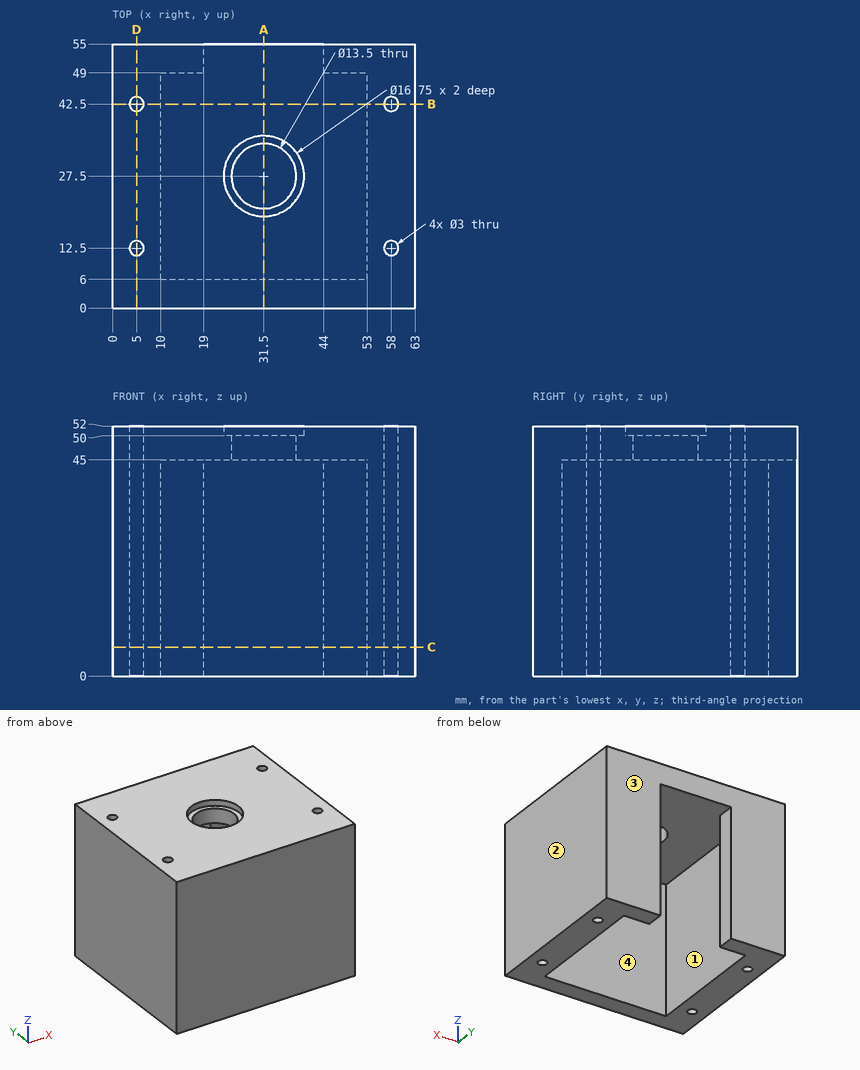
Here's the drawing with two shaded views (mm, measured from the low corner). I have some questions. Round coordinates to 2 decimals unless told otherwise and drop trailing zeros. Order: outer loops, then holes, each group sorted by start corner. A loop starts at its lowest first (then second) coordinate and runs counter-clockwise, first axis right, second up. Notation, with made-up numbers: (25, 72.5) -> (69, 72.5) arc R24 cw to (69, 109.5) -> close; hole circle Ø7 at (43, 34). An arc over 180 degrees is marked (long way). Use a Markdown table: item, result. Add a question column.
(1) Suppose I cut it at D-D, the plane x = 5. Please give me the cut outline in (y, z).
(2) Suppose I cut it at A-A, the plane x = 31.5. Please give me the cut outline in (y, z) (3 decimals).
(3) Suppose I cut it at B-B, the plane y = 42.5. Please give me the cut outline in (x, z).
(4) If we mould it in two halves opening along Y, with no side actions, what happens to the marked faces 1, 2, 3 and 4? For each: released by +Y, released by -Y, zero draft, split by the parting line, or undercut.
(5) For pin 1 Ø3.5 at (x, y) = (5, 42.5) entering from -Z; pin 2 Ø1.5 at (x, z) = (25, 36) entering from +Y; pin 3 Ø2.5 at (x, y) = (58, 12.5) entering from +Z; pin 4 Ø1.5 at (x, y) = (47, 11.5) entering from -Z, each with a flat end and sliding along its axis, tell me the tip position at first contact or that it passes through.
(6) I need wall thicknesses on line 1 along Y through (x, z) = (5, 19); line 2 along Y through (x, z) = (13.5, 24); line 3 along X through (y, z) = (48, 12). Which ranges of each line are inside material? Lowest first, please.
(7) Suppose I cut it at C-C, the plane z = 6. Please give me the cut outline in (x, y).
Verdict:
| question | item | result |
|---|---|---|
| 1 | outline | (0, 0) -> (11, 0) -> (11, 52) -> (0, 52) -> close; (14, 0) -> (41, 0) -> (41, 52) -> (14, 52) -> close; (44, 0) -> (55, 0) -> (55, 52) -> (44, 52) -> close |
| 2 | outline | (0, 0) -> (6, 0) -> (6, 45) -> (20.75, 45) -> (20.75, 50) -> (19.125, 50) -> (19.125, 52) -> (0, 52) -> close; (34.25, 45) -> (55, 45) -> (55, 52) -> (35.875, 52) -> (35.875, 50) -> (34.25, 50) -> close |
| 3 | outline | (0, 0) -> (3.5, 0) -> (3.5, 52) -> (0, 52) -> close; (6.5, 0) -> (10, 0) -> (10, 45) -> (53, 45) -> (53, 0) -> (56.5, 0) -> (56.5, 52) -> (6.5, 52) -> close; (59.5, 0) -> (63, 0) -> (63, 52) -> (59.5, 52) -> close |
| 4 | face 1 | undercut |
| 4 | face 2 | zero draft |
| 4 | face 3 | released by +Y |
| 4 | face 4 | undercut |
| 5 | pin 1 | z = 0 |
| 5 | pin 2 | y = 6 |
| 5 | pin 3 | through |
| 5 | pin 4 | z = 45 |
| 6 | line 1 | 0 to 11, 14 to 41, 44 to 55 |
| 6 | line 2 | 0 to 6, 49 to 55 |
| 6 | line 3 | 0 to 10, 53 to 63 |
| 7 | outline | (0, 0) -> (63, 0) -> (63, 55) -> (44, 55) -> (44, 49) -> (53, 49) -> (53, 6) -> (10, 6) -> (10, 49) -> (19, 49) -> (19, 55) -> (0, 55) -> close; hole circle Ø3 at (5, 12.5); hole circle Ø3 at (5, 42.5); hole circle Ø3 at (58, 12.5); hole circle Ø3 at (58, 42.5) |
